```python
from build123d import *

# Parameters (mm, degrees)
F1_R     = 6.75
F2_DEPTH = 15
F3_R     = 9
F4_DEPTH = 35
F5_W     = 35
F5_H     = 35
F5_R     = 9
F6_DEPTH = 6


with BuildPart() as f2:
    # F1 (on offset) → F2 (new body)
    with BuildSketch(Plane.XY.offset(40)):
        Circle(F1_R)
    extrude(amount=-F2_DEPTH)

    # F3 (on offset) → F4 (join)
    with BuildSketch(Plane.XY.offset(40)):
        Circle(F3_R)
    extrude(amount=F4_DEPTH)

    # F5 (on face) → F6 (join)
    with BuildSketch(Plane.XY.offset(75)):
        with Locations((0, -3.5)):
            Rectangle(F5_W, F5_H)
        Circle(F5_R, mode=Mode.SUBTRACT)
    extrude(amount=-F6_DEPTH)


solid = f2.part
```
CAD build for the part. Positions are in the model's coordinates, mm. A direction names the side the tool comes from. Round coordinates to 2 decimals unless told otherwise and drop trailing zeros. Loops run counter-clockwise (first coordinate to the right, second up) from the corner with the lowest first, then second, coordinate; pieces in that order, holes last. Notation, with made-up numbers: M 67.5,-19.75 L 73.5,-19.75 A16 ccw 73.5,6.25 Z; hole C 82.25,46.25 d11. An arc over 180 degrees is marked long. Use a Markdown table: item, result. Add a question column.
(1) Drill centre lines: line 1 (Z direction, x = 1, y = -17.5); line 2 (X direction, y = 0.5, z = 61.5); line 3 (Z direction, x = -5.5, y = 7). Where is each one in solid material? Low to high.
(2) Which spindle directions (+Z, -Z, +X, -X, +Y, -Y) get a long thin tool onto all of the face, cutting with end or side? Do faces 1 (the face through (-1.46, -6.59, 32.61)), 2 (the face through (0, -21, 72)). Say none if no direction does.
(3) Cut at A-A (y = 0). Give the cut face in (x, z).
(4) Cut at D-D (x = 8). Give the cut face in (y, z), and give its area (3 significant figures).
(5) Cut at C-C (z = 43). Give the cut face in (x, y).
(6) Flat gauge pins, fed straight in: pin 1 (12 mm diameter, centred on y = -1.5, z = 42, fed in from -X); pin 2 (1.5 mm diameter, centred on x = 4, z = 44.5, fed in from +Y); pin 3 (10 mm diameter, centred on x = -10, y = -12, fed in from -Z). Where does each tip first touch, or does it go through?
(7) Cut at B-B (x = 0). Give the cut face in (y, z).
Geometry says:
| question | item | result |
|---|---|---|
| 1 | line 1 | z = 69 to 75 |
| 1 | line 2 | x = -8.99 to 8.99 |
| 1 | line 3 | z = 40 to 75 |
| 2 | face 1 | -Z |
| 2 | face 2 | +Z, -Z, +X, -X, -Y |
| 3 | outline | M -17.5,69 L -9,69 L -9,40 L -6.75,40 L -6.75,25 L 6.75,25 L 6.75,40 L 9,40 L 9,69 L 17.5,69 L 17.5,75 L -17.5,75 Z |
| 4 | outline | M -21,69 L -4.12,69 L -4.12,40 L 4.12,40 L 4.12,69 L 14,69 L 14,75 L -21,75 Z |
| 4 | area | 449 mm² |
| 5 | outline | C 0,0 d18 |
| 6 | pin 1 | stops at x = -9 |
| 6 | pin 2 | stops at y = 8.39 |
| 6 | pin 3 | stops at z = 69 |
| 7 | outline | M -21,69 L -9,69 L -9,40 L -6.75,40 L -6.75,25 L 6.75,25 L 6.75,40 L 9,40 L 9,69 L 14,69 L 14,75 L -21,75 Z |
